Here's the drawing with two shaded views (mm, measured from the low corner). I have some questions. Give positions to 0.01 mm unless a question says otherwise; leave off trailing zeros. Loops run counter-clockwise (first coordinate to the right, second up) from the corner with the lowest first, then second, coordinate; pieces in that order, holes last.
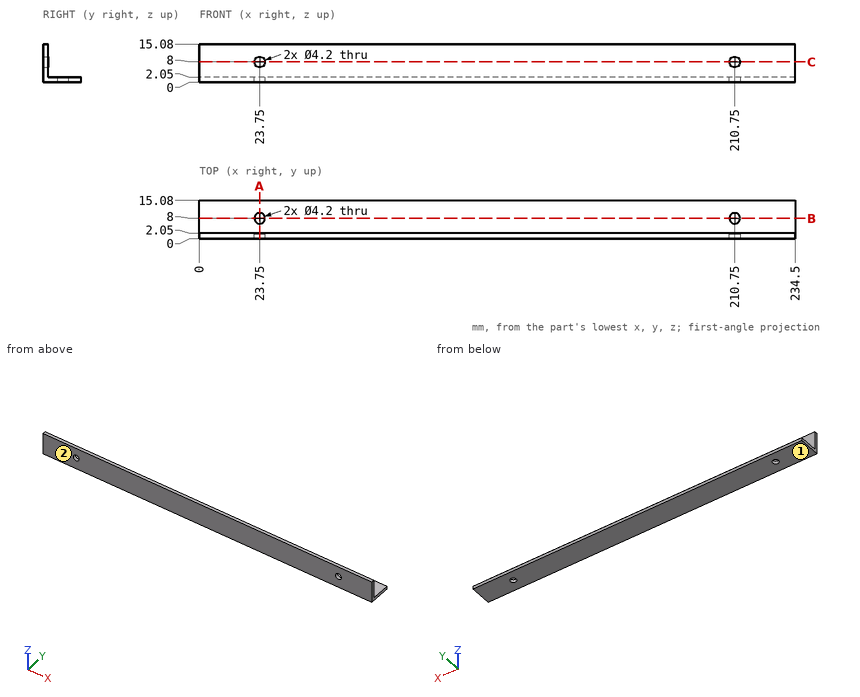
(1) Suppose I cut it at B-B on y = 8. List the corners of the cut face in (x, z) for me.
Returned:
outline: (0, 0) - (21.65, 0) - (21.65, 2.05) - (0, 2.05) - close; (25.85, 0) - (208.65, 0) - (208.65, 2.05) - (25.85, 2.05) - close; (212.85, 0) - (234.5, 0) - (234.5, 2.05) - (212.85, 2.05) - close
(2) Please list where these lines run through material, in increasing order: probe 1 along X at (y, z) = (1.6, 8); probe 2 along Y at (x, z) = (210.75, 1.2).
Returned:
probe 1: x = 0 to 21.65, 25.85 to 208.65, 212.85 to 234.5
probe 2: y = 0 to 5.9, 10.1 to 15.08
(3) Suppose I cut it at A-A on x = 23.75. List the corners of the cut face in (y, z) for me, plus the area to 3 significant figures.
Returned:
outline: (0, 0) - (5.9, 0) - (5.9, 2.05) - (2.05, 2.05) - (2.05, 5.9) - (0, 5.9) - close; (0, 10.1) - (2.05, 10.1) - (2.05, 15.08) - (0, 15.08) - close; (10.1, 0) - (15.08, 0) - (15.08, 2.05) - (10.1, 2.05) - close
area: 40.4 mm2
(4) Will these pins go through, and if not, where does the flat tip stop? P1, Ø2, axis at y = 3.5, z = 8.5, coming from the +X side; P2, Ø1.5, axis at x = 178.5, z = 10, coming from the +Y side.
Returned:
P1: passes through
P2: stops at y = 2.05
(5) Thinking about a two-plate mould opening in Z: for the marked faces 1 and 2, which applies, pulls with the +Z half, pulls with the -Z half, needs draft (parallel to the pull), parting line crosses it, or undercut?
Returned:
face 1: pulls with the -Z half
face 2: needs draft
